Geometry: final body of the model. Coordinates: model frame, mm. Face numbers are marked on the shaded views. A direction names the side the tool comes from. Give positions to 0.01 mm unless a question says otherwise; leave off trailing zeros. Write each loop counter-clockwise with the first axis right and the second up, starting at its lowest first coordinate (ties: lowest second). Pieces come first, ordered by that corner, then holes.
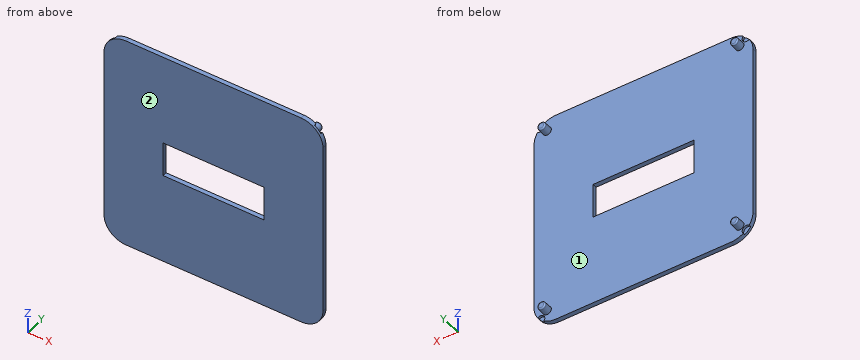
```python
from build123d import *

# Parameters (mm, degrees)
F0_W     = 46
F0_H     = 16
F1_DEPTH = 2
F2_R     = 1.9
F3_DEPTH = 4
F3_TAPER = 2
F5_DEPTH = 1
F6_R     = 0.6


# Not quite as in the source:
# - a feature names something its author has since deleted; it is built from what else it names


with BuildPart() as f1:
    # F0 (on Front) → F1 (new body)
    with BuildSketch(Plane.XZ):
        Polygon((-40, -50), (40, -50), (40, -40), (50, -40), (50, 40), (40, 40), (40, 50), (-40, 50), (-40, 40), (-50, 40), (-50, -40), (-40, -40), align=None)
        Rectangle(F0_W, F0_H, mode=Mode.SUBTRACT)
        with BuildLine():
            Line((40, -40), (40, -50))
            ThreePointArc((40, -50), (47.0710678119, -47.0710678119), (50, -40))
            Line((50, -40), (40, -40))
        make_face()
        with BuildLine():
            ThreePointArc((-50, -40), (-47.0710678119, -47.0710678119), (-40, -50))
            Line((-40, -50), (-40, -40))
            Line((-40, -40), (-50, -40))
        make_face()
        with BuildLine():
            Line((40, 40), (50, 40))
            ThreePointArc((50, 40), (47.0710678119, 47.0710678119), (40, 50))
            Line((40, 50), (40, 40))
        make_face()
        with BuildLine():
            ThreePointArc((-40, 50), (-47.0710678119, 47.0710678119), (-50, 40))
            Line((-50, 40), (-40, 40))
            Line((-40, 40), (-40, 50))
        make_face()
    extrude(amount=F1_DEPTH)

    # F2 (on face) → F3 (join)
    with BuildSketch(Plane(origin=(0, 0, 0), x_dir=(-1, 0, 0), z_dir=(0, 1, 0))):
        with Locations((-44, 44)):
            Circle(F2_R)
        with Locations((44, 44)):
            Circle(F2_R)
        with Locations((-44, -44)):
            Circle(F2_R)
        with Locations((44, -44)):
            Circle(F2_R)
    extrude(amount=F3_DEPTH, taper=F3_TAPER)

    # F4 (on face) → F5 (cut)
    with BuildSketch(Plane.XZ):
        with BuildLine():
            ThreePointArc((48.3367711836, 45.5225217277), (47.0710678119, 47.0710678119), (45.5225217277, 48.3367711836))
            ThreePointArc((45.5225217277, 48.3367711836), (45.6568542495, 45.6568542495), (48.3367711836, 45.5225217277))
        make_face()
        with BuildLine():
            ThreePointArc((-48.3367711836, 45.5225217277), (-45.6568542495, 45.6568542495), (-45.5225217277, 48.3367711836))
            ThreePointArc((-45.5225217277, 48.3367711836), (-47.0710678119, 47.0710678119), (-48.3367711836, 45.5225217277))
        make_face()
        with BuildLine():
            ThreePointArc((-48.3367711836, -45.5225217277), (-47.0710678119, -47.0710678119), (-45.5225217277, -48.3367711836))
            ThreePointArc((-45.5225217277, -48.3367711836), (-45.6568542495, -45.6568542495), (-48.3367711836, -45.5225217277))
        make_face()
        with BuildLine():
            ThreePointArc((48.3367711836, -45.5225217277), (45.6568542495, -45.6568542495), (45.5225217277, -48.3367711836))
            ThreePointArc((45.5225217277, -48.3367711836), (47.0710678119, -47.0710678119), (48.3367711836, -45.5225217277))
        make_face()
    extrude(amount=F5_DEPTH, mode=Mode.SUBTRACT)

    # F6
    f6_edges = [f1.edges().sort_by_distance(p)[0] for p in [
        (45.760317, 4, 44),
        (45.760317, 4, -44),
        (-42.239683, 4, 44),
        (-42.239683, 4, -44),
    ]]
    fillet(f6_edges, radius=F6_R)


solid = f1.part
```
Item 1: Section C-C, the plane y = 1. Return the cut outline in (x, z), plus the area to 3 significant figures.
Found:
outline: circle Ø3.73 at (-44, -44); circle Ø3.73 at (-44, 44); circle Ø3.73 at (44, -44); circle Ø3.73 at (44, 44)
area: 43.7 mm2
Item 2: Reachability of the marked faces 1 and 2 from +Z, -Z, +X, -X, +Y, -Y: full face, straight path, thin tool, end or side. Return the list, or none.
Found:
face 1: +Y
face 2: +Z, -Z, +X, -X, -Y
Item 3: Section D-D, the plane x = 24.5. Return the cut outline in (y, z).
Found:
outline: (-2, -50) - (0, -50) - (0, 50) - (-2, 50) - close
Item 4: Line query: L1, parallel to Z at x = -6, y = -0.75; L2, parallel to Y at x = 34, z = 41; L3, parallel to X at y = -0.5, z = -44. Output: solid intervals per line, ascending.
Found:
L1: z = -50 to -8, 8 to 50
L2: y = -2 to 0
L3: x = -49.17 to 49.17
Item 5: Section B-B, the plane z = -1.5. Return the cut outline in (x, y), plus the area to 3 significant figures.
Found:
outline: (-50, -2) - (-23, -2) - (-23, 0) - (-50, 0) - close; (23, -2) - (50, -2) - (50, 0) - (23, 0) - close
area: 108 mm2
Item 6: Section A-A, the plane x = -14. Return the cut outline in (y, z), plus the area to 3 significant figures.
Found:
outline: (-2, -50) - (0, -50) - (0, -8) - (-2, -8) - close; (-2, 8) - (0, 8) - (0, 50) - (-2, 50) - close
area: 168 mm2
Item 7: Pin query (flat end, axial travel): pin 1 Ø1 at (x, z) = (47.5, 47.5) entering from +Y; pin 2 Ø1.6 at (x, z) = (-47, 46.5) entering from +Y; pin 3 Ø1.5 at (x, z) = (27, 12.5) entering from +Y. Return the tip coordinate at first contact, or that it passes through.
Found:
pin 1: passes through
pin 2: stops at y = -1
pin 3: stops at y = 0
